Design review of the part built by this model. Coordinates are the model's own, in mm. A direction names the side the tool comes from. Coordinates: 2 decimals unless noted, no trailing zeros. Write each loop counter-clockwise with the first axis right and the second up, starting at its lowest first coordinate (ties: lowest second). Pieces come first, ordered by that corner, then holes. Notation, with made-up numbers: (6.25, 17) - (22.25, 17) arc R34 ccw to (22.25, 56) - close; hole circle Ø4 at (34, 87). An arc over 180 degrees is marked (long way). Answer as CSV lines item,"result". Start each with the question number.
Q1. For line 1 along X through (y, z) = (4, 31); line 2 along X through (y, z) = (-10, 11); line 3 along X through (y, z) = (-16.5, 18), list the stretches that pass through material, from the lowest coordinate up. Write a range as [from, to].
Q2. We need section C-C (y = -10). Write out the cut boundary in (x, z), plus the area to 3 significant figures.
Q3. We need section A-A (x = 0). Write out the cut boundary in (y, z) (3 decimals).
Q4. We need section D-D (z = 12). State how many separate pieces and enclosed holes the cut face has, plus the area to 3 significant figures.
Q5. Clearance check with flat-ended pins moving along their axes: pin 1 (10 mm diameter, centred on x = 7, z = 25, fed in from -Y); pin 2 (2 mm diameter, centred on x = -3, y = 19, fed in from +Z); pin 3 (10 mm diameter, centred on x = -13.5, z = 35.5, fed in from -Y). State where each tip first meets the part, or that it passes through.
Q6. Mouldability with a two-part tool opening along Y and no side actions: class faces 1 (the face through (22.1, 2.86, 19.72)), 2 (the face through (-0.364, -53.974, 19.72)), 3 (the face through (0, -33, 0)) as pulls with the +Y half, pulls with the -Y half, needs draft (parallel to the pull), parting line crosses it, or undercut.
Q7. Machinability: for faces 4 (the face through (0, 20, 15)), 5 (the face through (-22.14, 17.1, 19.72)), 6 (the face through (18.4, 18.96, 39.14)), which of the approach directions +Z, -Z, +X, -X, +Y, -Y give a long, thin tool a straight path to every point of the face, cutting with its end or side? Answer none if there is none.
from build123d import *

# Parameters (mm, degrees)
BOSS_EXTRUDE2_DEPTH     = 40
CUT_EXTRUDE1_DEPTH      = 72.681940717
CUT_EXTRUDE1_DEPTH_BACK = 72.681940717
SKETCH2_R               = 16
CUT_EXTRUDE3_DEPTH      = 72.681940717
FILLET1_R               = 3
SKETCH5_W               = 35
SKETCH5_H               = 15
CUT_EXTRUDE4_DEPTH      = 10
FILLET2_R               = 3


with BuildPart() as part:
    # Sketch1 → Boss-Extrude2 (new body)
    with BuildSketch(Plane.XY):
        with BuildLine():
            Line((-25, 0), (-25, -47.83618531))
            ThreePointArc((-25, -47.83618531), (0, -53.975), (25, -47.83618531))
            Line((25, -47.83618531), (25, 0))
            Line((25, 0), (25, 20))
            Line((25, 20), (-25, 20))
            Line((-25, 20), (-25, 0))
        make_face()
    extrude(amount=BOSS_EXTRUDE2_DEPTH)

    # Sketch2 → Cut-Extrude1 (cut, two sides: drawn at the far end of the back side and taken through both)
    with BuildSketch(Plane.XY.offset(40).offset(-CUT_EXTRUDE1_DEPTH_BACK)):
        with Locations((0, -10)):
            Circle(SKETCH2_R)
    extrude(amount=CUT_EXTRUDE1_DEPTH + CUT_EXTRUDE1_DEPTH_BACK, mode=Mode.SUBTRACT)

    # Sketch4 → Cut-Extrude3 (cut, through all)
    with BuildSketch(Plane.XY.offset(40)):
        with BuildLine():
            Line((-23, 18), (23, 18))
            Line((23, 18), (23, 2))
            Line((23, 2), (14.317821063, 2))
            ThreePointArc((14.317821063, 2), (0, 8.681541692), (-14.317821063, 2))
            Line((-14.317821063, 2), (-23, 2))
            Line((-23, 2), (-23, 18))
        make_face()
    extrude(amount=-CUT_EXTRUDE3_DEPTH, mode=Mode.SUBTRACT)

    # Fillet1
    fillet1_edges = [part.edges().sort_by_distance(p)[0] for p in [
        (23, 18, 20),
        (23, 2, 20),
        (14.317821063, 2, 20),
        (-14.317821063, 2, 20),
        (-23, 2, 20),
        (-23, 18, 20),
    ]]
    fillet(fillet1_edges, radius=FILLET1_R)

    # Sketch5 → Cut-Extrude4 (cut)
    with BuildSketch(Plane(origin=(0, 20, 0), x_dir=(1, 0, 0), z_dir=(0, 1, 0))):
        with Locations((0, -32.5)):
            Rectangle(SKETCH5_W, SKETCH5_H)
    extrude(amount=-CUT_EXTRUDE4_DEPTH, mode=Mode.SUBTRACT)

    # Fillet2
    fillet2_edges = [part.edges().sort_by_distance(p)[0] for p in [
        (17.5, 19, 40),
        (17.5, 19, 25),
        (-17.5, 19, 25),
        (-17.5, 19, 40),
    ]]
    fillet(fillet2_edges, radius=FILLET2_R)


solid = part.part
Results list:
1,line 1,"x = [-25, -22.83], [-12.37, -7.75], [7.75, 12.37], [22.83, 25]"
1,line 2,"x = [-25, -16], [16, 25]"
1,line 3,"x = [-25, -14.62], [14.62, 25]"
2,outline,"(-25, 0) - (-16, 0) - (-16, 40) - (-25, 40) - close; (16, 0) - (25, 0) - (25, 40) - (16, 40) - close"
2,area,"720 mm2"
3,outline,"(-53.975, 0) - (-26, 0) - (-26, 40) - (-53.975, 40) - close; (6, 0) - (8.682, 0) - (8.682, 40) - (6, 40) - close; (18, 0) - (20, 0) - (20, 25) - (18, 25) - close"
4,separate pieces,"1"
4,enclosed holes,"2"
4,area,"2,200 mm2"
5,pin 1,"stops at y = -53.94"
5,pin 2,"stops at z = 25"
5,pin 3,"stops at y = -53.3"
6,face 1,"undercut"
6,face 2,"pulls with the -Y half"
6,face 3,"needs draft"
7,face 4,"+Z, -Z, +X, -X, +Y"
7,face 5,"+Z, -Z"
7,face 6,"+Z, +Y"
